Model file for the job. Use its own axes, mm. Face numbers are marked on the shaded views. A direction names the side the tool comes from. Coordinates: 2 decimals unless noted, no trailing zeros. Write each loop counter-clockwise with the first axis right and the second up, starting at its lowest first coordinate (ties: lowest second). Pieces come first, ordered by that corner, then holes. Notation, with made-up numbers: M -0.75,-29.5 L 17.25,-29.5 A20 cw 17.25,-11.5 Z; hole C -33.75,-36 d7. An arc over 180 degrees is marked long. One line per question, with ' | ' between items. Start each with the question number.
(1) Cut at A-A (y = -16). Write the cut outline in (x, z) (3 decimals), plus the area to 3 significant figures.
(2) Tool access for the marked faces 1, 2 and 3: list every direction of +Z, -Z, +X, -X, +Y, -Y with a clear straight run to the whole face (end or side of a thin tool).
(3) Cut at B-B (x = 6). Write the cut outline in (y, z).
(4) Flat gauge pins, fed straight in: pin 1 Ø8 at (x, z) = (-5, 6.5) entering from -Y; pin 2 Ø8 at (y, z) = (14, 4.5) entering from +X; pin 3 Ø2 at (x, z) = (-14.5, 10) entering from +Y. Where does each tip first touch, or does it go through?
(5) Wall check: probe 1 along X at (y, z) = (-6, 7); probe 2 along X at (y, z) = (-5, 9.5); probe 3 along Y at (x, z) = (8.5, 11.5). Give the ranges that are in metal, low to high.
(6) Two-plate mould, pull along X, no slides. Class the marked faces 4, 5, 6 and 7: +X half, -X half, draft (parallel to the pull), parting line (faces both ways), or undercut.
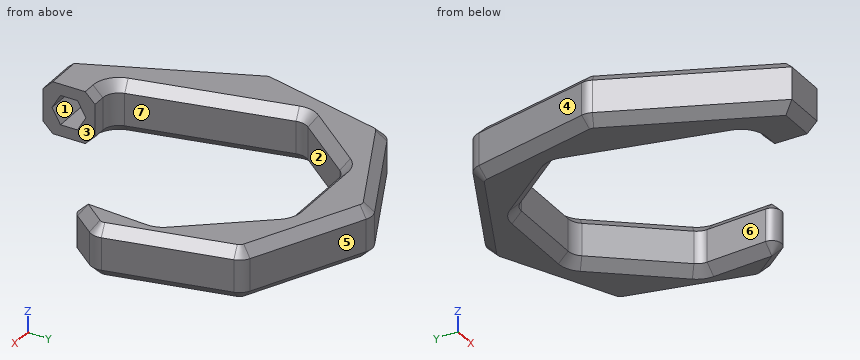
from build123d import *

# Parameters (mm, degrees)
F1_DEPTH = 16
F2_R     = 3
F3_R     = 5
F4_R     = 5
F5_W     = 16
F5_H     = 16
F6_DEPTH = 12
F7_DEPTH = 23
F8_SIZE  = 3


with BuildPart() as f1:
    # F0 (on Top) → F1 (new body)
    with BuildSketch(Plane.XY):
        Polygon((0, -61), (0, -45), (-20, -45), (-20.4101977074, -43.2465056593), (-20.8264194776, -43.2465056593), (-46.7965397847, -10.6810048299), (-25, -61), align=None)
        Polygon((-20.8264194776, -43.2465056593), (-20.4101977074, -43.2465056593), (-32.2850969664, 7.5157689065), (-46.7965397847, -10.6810048299), align=None)
        Polygon((-46.7965397847, -10.6810048299), (-32.2850969664, 7.5157689065), (-37.5279111585, 29.9275104892), align=None)
        Polygon((-37.5279111585, 29.9275104892), (-32.2850969664, 7.5157689065), (-14.4123294557, 29.9275104892), align=None)
        Polygon((0, 48), (-37.5279111585, 29.9275104892), (-14.4123294557, 29.9275104892), align=None)
        Polygon((0, 48), (-14.4123294557, 29.9275104892), (14.4123294557, 29.9275104892), align=None)
        Polygon((37.5279111585, 29.9275104892), (0, 48), (14.4123294557, 29.9275104892), align=None)
        Polygon((14.4123294557, 29.9275104892), (35.7777584033, 3.1361099918), (37.5279111585, 29.9275104892), align=None)
        Polygon((35.7777584033, 3.1361099918), (46.7965397847, -10.6810048299), (37.5279111585, 29.9275104892), align=None)
        Polygon((35.7777584033, 3.1361099918), (33.8114796312, -26.9637552446), (46.7965397847, -10.6810048299), align=None)
    extrude(amount=F1_DEPTH)

    # F2
    f2_edges = [f1.edges().sort_by_distance(p)[0] for p in [
        (33.81148, -26.963755, 8),
    ]]
    fillet(f2_edges, radius=F2_R)

    # F3
    f3_edges = [f1.edges().sort_by_distance(p)[0] for p in [
        (-46.79654, -10.681005, 8),
        (-37.527911, 29.92751, 8),
        (0, 48, 8),
        (37.527911, 29.92751, 8),
        (46.79654, -10.681005, 8),
    ]]
    fillet(f3_edges, radius=F3_R)

    # F4
    f4_edges = [f1.edges().sort_by_distance(p)[0] for p in [
        (-32.285097, 7.515769, 8),
        (-14.412329, 29.92751, 8),
        (14.412329, 29.92751, 8),
        (35.777758, 3.13611, 8),
        (-20, -45, 8),
    ]]
    fillet(f4_edges, radius=F4_R)

    # F5 (on face) → F6 (cut)
    with BuildSketch(Plane.YZ):
        with Locations((-53, 8)):
            Rectangle(F5_W, F5_H)
        Polygon((-50.3874900319, 3.475), (-55.6125099681, 3.475), (-58.2250199362, 8), (-55.6125099681, 12.525), (-50.3874900319, 12.525), (-47.7749800638, 8), align=None, mode=Mode.SUBTRACT)
        Polygon((-58.2250199362, 8), (-55.6125099681, 3.475), (-50.3874900319, 3.475), (-47.7749800638, 8), (-50.3874900319, 12.525), (-55.6125099681, 12.525), align=None)
    extrude(amount=-F6_DEPTH, mode=Mode.SUBTRACT)

    # F5 (on face) → F7 (cut)
    with BuildSketch(Plane.YZ):
        Polygon((-58.2250199362, 8), (-55.6125099681, 3.475), (-50.3874900319, 3.475), (-47.7749800638, 8), (-50.3874900319, 12.525), (-55.6125099681, 12.525), align=None)
    extrude(amount=-F7_DEPTH, mode=Mode.SUBTRACT)

    # F8
    f8_edges = [f1.edges().sort_by_distance(p)[0] for p in [
        (-26.318032, -17.991965, 16),
        (-18.5, -61, 16),
        (-18.5, -61, 0),
        (-26.318032, -17.991965, 0),
    ]]
    chamfer(f8_edges, length=F8_SIZE)


solid = f1.part
Filled in:
1) outline: M -44.493,3 L -41.223,0 L -29.865,0 L -26.784,3 L -26.784,13 L -29.865,16 L -41.223,16 L -44.493,13 Z; M 34.528,3 L 37.534,0 L 38.718,0 L 42.555,3 L 42.555,13 L 38.718,16 L 37.534,16 L 34.528,13 Z | area: 372 mm²
2) face 1: +X | face 2: +Z, -Z | face 3: +Z, -Z, +X, -Y
3) outline: M 29.93,3 L 32.93,0 L 41.78,0 L 45.11,3 L 45.11,13 L 41.78,16 L 32.93,16 L 29.93,13 Z
4) pin 1: y = 29.93 | pin 2: x = 42.08 | pin 3: y = 41.5
5) probe 1: -45.73 to -29.12, 35.18 to 45.73 | probe 2: -45.5 to -29.36, 35.25 to 45.5 | probe 3: 29.93 to 43.91
6) face 4: -X half | face 5: +X half | face 6: undercut | face 7: undercut
